```python
from build123d import *

# Parameters (mm, degrees)
EXTRUDE_1_DEPTH     = 2.5
SKETCH_2_W          = 15.8
SKETCH_2_H          = 6.5
EXTRUDE_2_DEPTH     = 1
FILLET_1_R          = 0.5
CUT_EXTRUDE_1_DEPTH = 12.419391402
SKETCH_4_W          = 12.1
SKETCH_4_H          = 6.5
CUT_EXTRUDE_2_DEPTH = 11.932177276
FILLET_2_R          = 0.5
CHAMFER_1_SIZE      = 0.5


with BuildPart() as part:
    # 草图1 → 凸台-拉伸1 (new body)
    with BuildSketch(Plane.XY):
        with BuildLine():
            Line((-9.05, -1.25), (-9.05, -3.45))
            ThreePointArc((-9.05, -3.45), (-8.713172798, -4.263172798), (-7.9, -4.6))
            Line((-7.9, -4.6), (7.9, -4.6))
            ThreePointArc((7.9, -4.6), (8.713172798, -4.263172798), (9.05, -3.45))
            Line((9.05, -3.45), (9.05, -1.25))
            ThreePointArc((9.05, -1.25), (8.713172798, -0.436827202), (7.9, -0.1))
            Line((7.9, -0.1), (-7.9, -0.1))
            ThreePointArc((-7.9, -0.1), (-8.713172798, -0.436827202), (-9.05, -1.25))
        make_face()
    extrude(amount=-EXTRUDE_1_DEPTH)

    # 草图2 → 凸台-拉伸2 (add)
    with BuildSketch(Plane(origin=(0, 0, -2.5), x_dir=(-1, 0, 0), z_dir=(0, 0, -1))):
        with Locations((0, -2.35)):
            Rectangle(SKETCH_2_W, SKETCH_2_H)
    extrude(amount=-EXTRUDE_2_DEPTH)

    # 圆角1
    fillet_1_edges = [part.edges().sort_by_distance(p)[0] for p in [
        (-7.9, 0.9, -2),
        (-7.9, -5.6, -2),
        (7.9, -5.6, -2),
        (7.9, 0.9, -2),
    ]]
    fillet(fillet_1_edges, radius=FILLET_1_R)

    # 草图3 → 切除-拉伸1 (cut, through all)
    with BuildSketch(Plane(origin=(0, 0.9, 0), x_dir=(1, 0, 0), z_dir=(0, 1, 0))):
        Polygon((8.475, 2.5), (9.05, 1.925), (9.05, 2.5), align=None)
        Polygon((-9.05, 1.925), (-9.05, 2.5), (-8.475, 2.5), align=None)
    extrude(amount=-CUT_EXTRUDE_1_DEPTH, mode=Mode.SUBTRACT)

    # 草图4 → 切除-拉伸2 (cut, through all)
    with BuildSketch(Plane(origin=(0, 0, -2.5), x_dir=(-1, 0, 0), z_dir=(0, 0, -1))):
        with Locations((3, -2.35)):
            Rectangle(SKETCH_4_W, SKETCH_4_H)
    extrude(amount=-CUT_EXTRUDE_2_DEPTH, mode=Mode.SUBTRACT)

    # 圆角2
    fillet_2_edges = [part.edges().sort_by_distance(p)[0] for p in [
        (3.05, -4.6, -0.75),
        (3.05, -0.1, -0.75),
        (3.05, 0.9, -2),
        (3.05, -5.6, -2),
    ]]
    fillet(fillet_2_edges, radius=FILLET_2_R)

    # 倒角1
    chamfer_1_edges = [part.edges().sort_by_distance(p)[0] for p in [
        (3.05, -2.35, 0),
        (5.725, -4.6, 0),
        (3.196446609, -0.246446609, 0),
        (3.196446609, -4.453553391, 0),
        (5.725, -0.1, 0),
        (8.713172798, -0.436827202, 0),
        (9.05, -2.35, 0),
        (8.713172798, -4.263172798, 0),
    ]]
    chamfer(chamfer_1_edges, length=CHAMFER_1_SIZE - 0.0001)  # a hair under: the kernel refuses the full size


solid = part.part
```
Geometry check sheet. Reference: the model listing, model coordinates, mm. A direction names the side the tool comes from. Give positions to 0.01 mm unless a question says otherwise; leave off trailing zeros. Order: outer loops, then holes, each group sorted by start corner. A loop starts at its lowest first (then second) coordinate and runs counter-clockwise, first axis right, second up. Notation, with made-up numbers: (66, 53.25) -> (111, 53.25) arc R24 cw to (111, 83.25) -> close; hole circle Ø10 at (66, -23.75). An arc over 180 degrees is marked (long way). Write each question's results on one line, items separated by ' | '. Start each with the question number.
(1) Access from +Z, -Z, +X, -X, +Y, -Y to the whole of each face (thin tool, end or side, straight path). Record for faces 1 (the face through (8.722, -0.446, -1.486)), 2 (the face through (6, -0.1, -1)).
(2) Sectioned sample at C-C (y = -1.5). Enter the section's corners in (x, z) (3 decimals).
(3) Scan lines: line 1 (Y direction, x = 6, z = -0.8); line 2 (Z direction, x = 7.75, y = -0.5); line 3 (Z direction, x = 7.5, y = 0.5). Record each from-to range of solid material in increasing order.
(4) Sectioned sample at D-D (z = -1.6). Enter the section's corners in (x, y), plus the area to 3 significant figures.
(5) Gauge pin test, flat ends, axial feed: P1, Ø0.6, axis at y = 0, z = -2, coming from the +X side; P2, Ø1.6, axis at x = 4.5, y = 0.5, coming from the +Z side; P3, Ø0.8, axis at x = 6, z = -1, coming from the -Y side. Record the tip position at first contact, or that the pin passes through.
(6) Sectioned sample at B-B (x = 7). Enter the section's corners in (y, z).
(7) Mould release check, pull along Y, two halves, no side actions. Record for faces 3 (the face through (5.5, 0.3, -1.5)), 4 (the face through (6, -4.6, -1)), 5 (the face through (6, 0.9, -2)): pulls with the +Y half, pulls with the -Y half, needs draft (parallel to the pull), parting line crosses it, or undercut.
(8) Sectioned sample at A-A (z = -0.75). Enter the section's corners in (x, y), plus the area to 3 significant figures.
Answer below:
1) face 1: +Z, -Z, +X, +Y | face 2: +Z, +X, -X, +Y
2) outline: (3.05, -2.5) -> (8.475, -2.5) -> (9.05, -1.925) -> (9.05, -0.5) -> (8.55, 0) -> (3.55, 0) -> (3.05, -0.5) -> close
3) line 1: -4.6 to -0.1 | line 2: -2.5 to -0.1 | line 3: -2.5 to -1.5
4) outline: (3.05, -5.1) arc R0.5 ccw to (3.55, -5.6) -> (7.4, -5.6) arc R0.5 ccw to (7.9, -5.1) -> (7.9, -4.6) arc R1.15 ccw to (9.05, -3.45) -> (9.05, -1.25) arc R1.15 ccw to (7.9, -0.1) -> (7.9, 0.4) arc R0.5 ccw to (7.4, 0.9) -> (3.55, 0.9) arc R0.5 ccw to (3.05, 0.4) -> close | area: 35.9 mm2
5) P1: x = 8.55 | P2: z = -0.3 | P3: y = -4.6
6) outline: (-5.6, -2.5) -> (0.9, -2.5) -> (0.9, -1.5) -> (-0.1, -1.5) -> (-0.1, -0.5) -> (-0.6, 0) -> (-4.1, 0) -> (-4.6, -0.5) -> (-4.6, -1.5) -> (-5.6, -1.5) -> close
7) face 3: needs draft | face 4: pulls with the -Y half | face 5: pulls with the +Y half
8) outline: (3.05, -4.1) arc R0.5 ccw to (3.55, -4.6) -> (7.9, -4.6) arc R1.15 ccw to (9.05, -3.45) -> (9.05, -1.25) arc R1.15 ccw to (7.9, -0.1) -> (3.55, -0.1) arc R0.5 ccw to (3.05, -0.6) -> close | area: 26.3 mm2
